The model under review builds one solid part; all positions refer to its coordinate system, in mm. A direction names the side the tool comes from. Give positions to 0.01 mm unless a question says otherwise; leave off trailing zeros. Order: outer loops, then holes, each group sorted by start corner. A loop starts at its lowest first (then second) coordinate and runs counter-clockwise, first axis right, second up.
Autodesk Inventor part; units mm, degrees
ref_plane "YZ Plane" through (0, 0, 0) normal (1, 0, 0) x (0, 1, 0)
ref_plane "XZ Plane" through (0, 0, 0) normal (0, 1, 0) x (-1, 0, 0)
ref_plane "XY Plane" through (0, 0, 0) normal (0, 0, 1) x (1, 0, 0)
sketch "Sketch1" plane through (0, 0, 0) normal (0, 1, 0) x (-1, 0, 0)
  line L0 (0, 0) -> (0, 130)
  line L1 (0, 130) -> (0.5, 130)
  line L2 (0.5, 130) -> (0.5, 0.5)
  line L3 (0.5, 0.5) -> (32, 0.5)
  line L4 (32, 0.5) -> (32, 0)
  line L5 (32, 0) -> (0, 0)
  dimension "d0" = 0.5
  dimension "d1" = 130
  dimension "d2" = 32
extrude "Extrusion1" add sketch "Sketch1" along normal mid plane 100
sketch "Sketch2" plane through (0, -50, 0) normal (1, 0, 0) x (0, 0, -1)
  line L0 (-116.2978, 40.4754) -> (-102.0897, 40.4754)
  line L1 (-102.0897, 40.4754) -> (-102.0897, 56.9569)
  line L2 (-102.0897, 56.9569) -> (-116.2978, 56.9569)
  line L3 (-116.2978, 56.9569) -> (-116.2978, 40.4754)
  line L4 (-116.2978, -0.6285) -> (-92.269, -0.6285)
  line L5 (-92.269, -0.6285) -> (-92.269, 13.8246)
  line L6 (-92.269, 13.8246) -> (-116.2978, 13.8246)
  line L7 (-116.2978, 13.8246) -> (-116.2978, -0.6285)
  line L8 (-68.5175, -0.6285) -> (-43.5049, -0.6285)
  line L9 (-43.5049, -0.6285) -> (-43.5049, 14.8755)
  line L10 (-43.5049, 14.8755) -> (-68.5175, 14.8755)
  line L11 (-68.5175, 14.8755) -> (-68.5175, -0.6285)
  line L12 (-116.2978, 101.3011) -> (-92.269, 101.3011)
  line L13 (-92.269, 101.3011) -> (-92.269, 87.6013)
  line L14 (-92.269, 87.6013) -> (-116.2978, 87.6013)
  line L15 (-116.2978, 87.6013) -> (-116.2978, 101.3011)
  line L16 (-33.7527, 25.6785) -> (-78.3542, 25.6785) construction
  line L17 (-33.7527, 23.1785) -> (-78.3542, 23.1785)
  line L18 (-78.3542, 28.1785) -> (-33.7527, 28.1785)
  arc A0 (-33.7527, 23.1785) -> (-33.7527, 28.1785) centre (-33.7527, 25.6785) ccw
  arc A1 (-78.3542, 28.1785) -> (-78.3542, 23.1785) centre (-78.3542, 25.6785) ccw
  line L19 (-33.7526, 62.8674) -> (-78.3542, 62.8674) construction
  line L20 (-33.7526, 65.3674) -> (-78.3542, 65.3674)
  line L21 (-78.3542, 60.3674) -> (-33.7526, 60.3674)
  arc A2 (-33.7526, 60.3674) -> (-33.7526, 65.3674) centre (-33.7526, 62.8674) ccw
  arc A3 (-78.3542, 65.3674) -> (-78.3542, 60.3674) centre (-78.3542, 62.8674) ccw
  line L22 (-76.0973, 50.4436) -> (-80.6111, 75.2913) construction
  line L23 (-73.3501, 50.9427) -> (-77.8639, 75.7903)
  line L24 (-83.3583, 74.7922) -> (-78.8445, 49.9445)
  arc A4 (-78.8445, 49.9445) -> (-73.3501, 50.9427) centre (-76.0973, 50.4436) ccw
  arc A5 (-77.8639, 75.7903) -> (-83.3583, 74.7922) centre (-80.6111, 75.2913) ccw
  line L25 (-75.2925, 37.1839) -> (-81.416, 14.1731) construction
  line L26 (-78.3502, 37.9976) -> (-84.4737, 14.9868)
  line L27 (-78.3582, 13.3594) -> (-72.2347, 36.3702)
  arc A6 (-72.2347, 36.3702) -> (-78.3502, 37.9976) centre (-75.2925, 37.1839) ccw
  arc A7 (-84.4737, 14.9868) -> (-78.3582, 13.3594) centre (-81.416, 14.1731) ccw
  point P0 (0, 50)
  point P1 (-56.0534, 25.6785)
  point P2 (-56.0534, 62.8674)
  dimension "d16" = 2.5
extrude "Extrusion2" cut sketch "Sketch2" against normal blind 100
sketch "Sketch5" plane through (-32, 50, 0.5) normal (0, 0, 1) x (1, 0, 0)
  line L0 (6.4118, -5.271) -> (6.4118, -44.3585) construction
  line L1 (4.397, -5.271) -> (4.397, -44.3585)
  line L2 (8.4266, -44.3585) -> (8.4266, -5.271)
  arc A0 (8.4266, -5.271) -> (4.397, -5.271) centre (6.4118, -5.271) ccw
  arc A1 (4.397, -44.3585) -> (8.4266, -44.3585) centre (6.4118, -44.3585) ccw
  line L3 (6.4118, -53.8282) -> (6.4118, -93.3186) construction
  line L4 (4.397, -53.8282) -> (4.397, -93.3186)
  line L5 (8.4266, -93.3186) -> (8.4266, -53.8282)
  arc A2 (8.4266, -53.8282) -> (4.397, -53.8282) centre (6.4118, -53.8282) ccw
  arc A3 (4.397, -93.3186) -> (8.4266, -93.3186) centre (6.4118, -93.3186) ccw
  line L6 (16.7722, -25.4192) -> (16.7722, -5.271) construction
  line L7 (14.9589, -25.4192) -> (14.9589, -5.271)
  line L8 (18.5856, -5.271) -> (18.5856, -25.4192)
  arc A4 (14.9589, -25.4192) -> (18.5856, -25.4192) centre (16.7722, -25.4192) ccw
  arc A5 (18.5856, -5.271) -> (14.9589, -5.271) centre (16.7722, -5.271) ccw
  line L9 (16.7722, -73.5734) -> (16.7722, -93.3186) construction
  line L10 (15.3955, -73.5734) -> (15.3955, -93.3186)
  line L11 (18.1489, -93.3186) -> (18.1489, -73.5734)
  arc A6 (18.1489, -73.5734) -> (15.3955, -73.5734) centre (16.7722, -73.5734) ccw
  arc A7 (15.3955, -93.3186) -> (18.1489, -93.3186) centre (16.7722, -93.3186) ccw
  line L12 (28.3587, -63.1068) -> (21.2143, -63.1068)
  line L13 (21.2143, -63.1068) -> (21.2143, -77.826)
  line L14 (21.2143, -77.826) -> (28.3587, -77.826)
  line L15 (28.3587, -77.826) -> (28.3587, -73.5734)
  line L16 (28.3587, -73.5734) -> (24.1409, -73.5734)
  line L17 (24.1409, -73.5734) -> (24.1409, -67.3246)
  line L18 (24.1409, -67.3246) -> (28.3587, -67.3246)
  line L19 (28.3587, -67.3246) -> (28.3587, -63.1068)
  point P0 (32, -50)
  point P1 (6.4118, -24.8148)
  point P2 (6.4118, -73.5734)
  point P3 (16.7722, -15.3451)
  point P4 (16.7722, -83.446)
extrude "Extrusion5" cut sketch "Sketch5" against normal blind 10
properties part number "Platina lateral interna 2" material "Steel"
Item 1: Clearance check with flat-ended pins moving along their axes: pin 1 Ø0.6 at (x, z) = (0, 101) entering from +Y; pin 2 Ø1.5 at (x, y) = (-10.5, 11) entering from +Z; pin 3 Ø2 at (y, z) = (-27.5, 92.5) entering from -X. State where each tip first meets the part, or that it passes through.
Values found:
pin 1: stops at y = 37.6
pin 2: stops at z = 0.5
pin 3: stops at x = -0.5
Item 2: Take a section at D-D (z = 96). Give the boundary of the cut face in (x, y), and give its area (3 significant figures).
Values found:
outline: (-0.5, -36.18) - (0, -36.18) - (0, 37.6) - (-0.5, 37.6) - close
area: 36.9 mm2
Item 3: Take a section at A-A (z = 48). Give the boundary of the cut face in (x, y).
Values found:
outline: (-0.5, -35.12) - (0, -35.12) - (0, -26.82) - (-0.5, -26.82) - close; (-0.5, -21.82) - (0, -21.82) - (0, 10.37) - (-0.5, 10.37) - close; (-0.5, 15.37) - (0, 15.37) - (0, 50) - (-0.5, 50) - close
Item 4: Take a section at B-B (y = 43). Give the boundary of the cut face in (x, z), and give its area (3 significant figures).
Values found:
outline: (-32, 0) - (-27.6, 0) - (-27.6, 0.5) - (-32, 0.5) - close; (-23.57, 0) - (-17.04, 0) - (-17.04, 0.5) - (-23.57, 0.5) - close; (-13.41, 0) - (0, 0) - (0, 92.27) - (-0.5, 92.27) - (-0.5, 0.5) - (-13.41, 0.5) - close; (-0.5, 116.3) - (0, 116.3) - (0, 130) - (-0.5, 130) - close
area: 64.9 mm2
Item 5: Take a section at C-C (x = -25). Give the boundary of the cut face in (y, z).
Values found:
outline: (-50, 0) - (-45.25, 0) - (-45.25, 0.5) - (-50, 0.5) - close; (-1.9, 0) - (3.71, 0) - (3.71, 0.5) - (-1.9, 0.5) - close; (46.66, 0) - (50, 0) - (50, 0.5) - (46.66, 0.5) - close
Item 6: For faces 5 (the flat face through (0, -1, 64)), 6 (the flat face through (-0.246, 12.542, 81.133)), 7 (the flat face through (-0.5, -1, 66)), list the 3-axis set-ups (+Z, -Z, +X, -X, +Y, -Y) from which the entire face can be reached by the end or side of a thin tool; tool diameter is ignored.
Values found:
face 5: +Z, -Z, +X, +Y, -Y
face 6: +X, -X
face 7: +Z, -X, +Y, -Y
Item 7: For line 1 (Z direction, x = -5.5, y = 44); line 2 (X direction, y = 19.5, z = 103), list the stretches that pass through material, from the lowest coordinate up.
Values found:
line 1: z = 0 to 0.5
line 2: x = -0.5 to 0
Item 8: Draft analysis for pull direction Z (two halves, no side actions). For faces 1 (the flat face through (-16, -1, 0.5)), 2 (the flat face through (-16, -1, 0)), 3 (the cylindrical face through (-0.246, -2.314, 75.659)), 4 (the cylindrical face through (-0.25, 28.05, 81.05)), state which applies: released by +Z, released by -Z, zero draft, split by the parting line, or undercut.
Values found:
face 1: released by +Z
face 2: released by -Z
face 3: undercut
face 4: undercut
